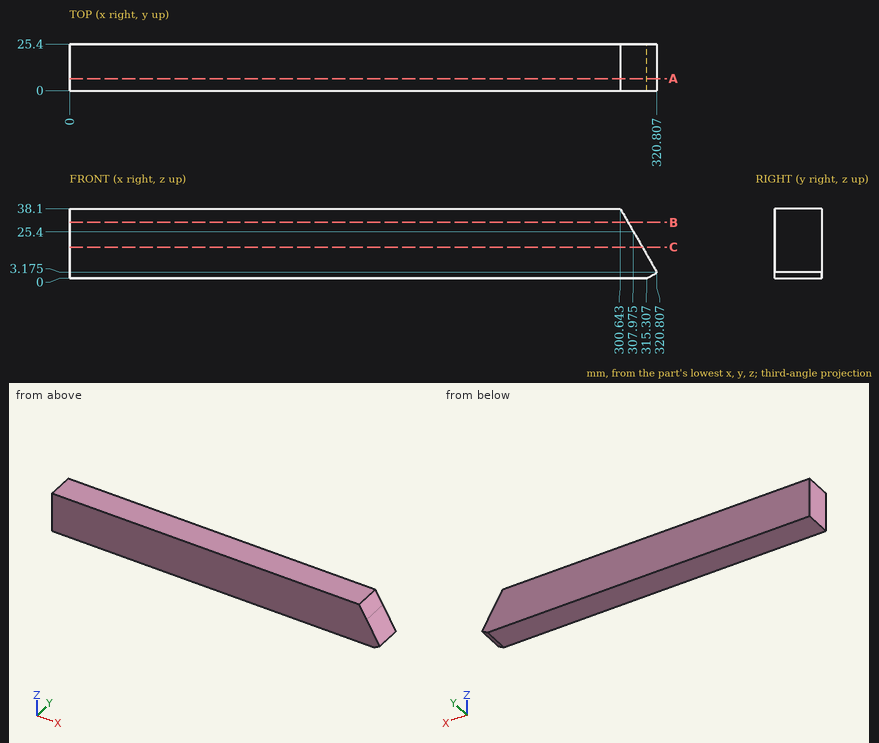
Job drawing, mm, ordinate dimensions from the low corner. One solid piece. Give positions to 0.01 mm unless a question says otherwise; leave off trailing zeros. Write each loop counter-clockwise with the first axis right and the second up, starting at its lowest first coordinate (ties: lowest second). Pieces come first, ordered by that corner, then holes. Notation, with made-up numbers: (-4.5, -23) - (0.5, -23) arc R6 cw to (0.5, -17) - close; hole circle Ø3 at (36, -4). An arc over 180 degrees is marked (long way). Use one line per item in the form item = value. Start each with the question number.
1. Band-saw the part on B-B on z = 30.5. Write the cut outline in (x, y), plus the area to 3 significant figures.
2. Band-saw the part on C-C on z = 17. Write the cut outline in (x, y) (1 decimal).
3. Drop flat-ended pins along their axis: pin 1 Ø1.5 at (y, z) = (9, 33.5) entering from +X; pin 2 Ø3 at (y, z) = (6.5, 29) entering from +X; pin 3 Ø5 at (y, z) = (19, 27.5) entering from +X (1 decimal). Give the stop position or say it passes through.
4. Band-saw the part on A-A on y = 6.5. Write the cut outline in (x, z) (1 decimal).
5. Probe line 1 (X direction, y = 7, z = 22.5); line 2 (X direction, y = 17.25, z = 21.5) (1 decimal). List the from-to ranges inside material, lowest first. Write a range as [from, to].
Conclusion:
q1.outline = (0, 0) - (305.03, 0) - (305.03, 25.4) - (0, 25.4) - close
q1.area = 7,750 mm²
q2.outline = (0, 0) - (312.8, 0) - (312.8, 25.4) - (0, 25.4) - close
q3.pin_1 = 303.73
q3.pin_2 = 306.76
q3.pin_3 = 308.2
q4.outline = (0, 0) - (315.3, 0) - (320.8, 3.2) - (300.6, 38.1) - (0, 38.1) - close
q5.line_1 = [0, 309.65]
q5.line_2 = [0, 310.2]
